Read the model definition and answer for the solid it produces. Units are mm, in the model's axes. Face numbers are marked on the shaded views. A direction names the side the tool comes from. Give positions to 0.01 mm unless a question says otherwise; leave off trailing zeros. Order: outer loops, then holes, each group sorted by start corner. A loop starts at its lowest first (then second) coordinate and runs counter-clockwise, first axis right, second up. Notation, with made-up numbers: M 84,54 L 113,54 A18 ccw 113,79 Z; hole C 65.25,2 d8. An arc over 180 degrees is marked long. One line per item, written item: value.
Autodesk Inventor part; units mm, degrees
ref_plane "YZ Plane" through (0, 0, 0) normal (1, 0, 0) x (0, 1, 0)
ref_plane "XZ Plane" through (0, 0, 0) normal (0, 1, 0) x (-1, 0, 0)
ref_plane "XY Plane" through (0, 0, 0) normal (0, 0, 1) x (1, 0, 0)
sketch "Sketch5" plane through (0, 0, 0) normal (0, 0, 1) x (1, 0, 0)
  line L0 (52.5, -15.6) -> (52.5, -10.6)
  line L1 (52.5, -10.6) -> (50, -10.6)
  line L2 (50, -10.6) -> (50, -12.625)
  line L3 (44, -12.625) -> (44, -2.975)
  line L4 (50, -2.975) -> (50, -5)
  line L5 (50, -5) -> (52.5, -5)
  line L6 (52.5, -5) -> (52.5, 0)
  line L7 (52.5, 0) -> (7.8, 0)
  line L8 (44, -2.975) -> (50, -2.975)
  line L9 (44, -12.625) -> (50, -12.625)
  line L10 (52.5, -15.6) -> (7.8, -15.6)
  line L11 (7.8, -15.6) -> (0, -15.6)
  line L12 (0, -15.6) -> (0, 0)
  line L13 (0, 0) -> (7.8, 0)
  point P0 (7.8, 0)
  dimension "d41" = 6
  dimension "d48" = 44
  dimension "d50" = 2.5
  dimension "d63" = 44.7
  dimension "d71" = 0
  dimension "d87" = 5.6
  dimension "d88" = 9.65
  dimension "d97" = 15.6
extrude "Extrusion2" add sketch "Sketch5" along normal blind 12
fillet "Fillet2" radius 15 1 edges at (0, -15.6, 6)
sketch "Sketch11" plane through (0, 0, 12) normal (0, 0, 1) x (1, 0, 0)
  line L0 (44, -2.975) -> (50, -2.975)
  circle A0 centre (44, -2.975) radius 0.5
  line L1 (44, -12.625) -> (44, -2.975)
  circle A1 centre (44, -12.625) radius 0.5
  line L2 (50, -12.625) -> (44, -12.625)
  circle A2 centre (50, -12.625) radius 0.5
  line L3 (50, -2.975) -> (50, -5)
  circle A3 centre (50, -2.975) radius 0.5
  point P0 (0, 0)
  dimension "d99" = 1
  dimension "d100" = 1
  dimension "d101" = 1
  dimension "d102" = 1
extrude "Extrusion7" cut sketch "Sketch11" against normal through all
fillet "Rundung3" radius 5 1 edges at (0, 0, 6)
equation "\"l1\" = 8"
properties part number "Maria_Greifer_3D-Druck"
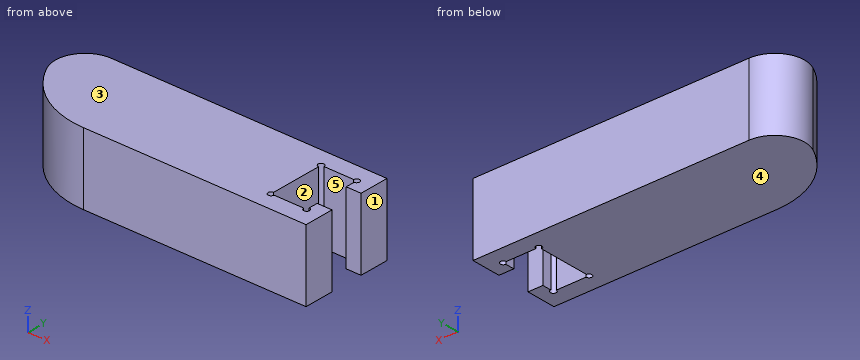
1) Which of the six approach directions +Z, -Z, +X, -X, +Y, -Y give full straight-line access (tool end or side, diameter ignored) to the marked faces 4 and 5?
Reported:
face 4: -Z, +X, -X, +Y, -Y
face 5: +Z, -Z
2) Determine the mould class of the marked faces 1, 2 and 3 for opening direction X: +X half, -X half, draft (parallel to the pull), parting line (faces both ways), or undercut.
Reported:
face 1: +X half
face 2: undercut
face 3: draft
3) Consider probe 1 along X at (y, z) = (-4.75, 8.5); probe 2 along X at (y, z) = (-11, 10.5); probe 3 along X at (y, z) = (-0.75, 2.25). Determine where each line is inside the solid, lowest interval first.
Reported:
probe 1: x = 1.03 to 44, 50 to 52.5
probe 2: x = 4.19 to 44, 50 to 52.5
probe 3: x = 3.39 to 52.5
4) Each of these flat-tipped pins is pushed along its axis until it touches: pin 1 Ø2 at (x, y) = (41.5, -11) entering from -Z; pin 2 Ø0.5 at (y, z) = (-11, 8.5) entering from -X; pin 3 Ø1 at (y, z) = (-4, 2) entering from -X. Where does it stop, or does it pass through?
Reported:
pin 1: stops at z = 0
pin 2: stops at x = 3.96
pin 3: stops at x = 1.05
5) Find section A-A, the plane x = 49. Write down the section's boundary in (y, z) (3 decimals).
Reported:
outline: M -15.6,0 L -12.625,0 L -12.625,12 L -15.6,12 Z; M -2.975,0 L 0,0 L 0,12 L -2.975,12 Z
